Here's how the part is built. I have some questions about the finished solid (model axes, mm). Coordinates: 2 decimals unless noted, no trailing zeros. Write each loop counter-clockwise with the first axis right and the second up, starting at its lowest first coordinate (ties: lowest second). Pieces come first, ordered by that corner, then holes.
Item 1: If we section it at B-B (x = 35): Please give me the cut outline in (y, z).
Item 2: If I drill on line 1 (Y direction, x = 61, z = 51); line 2 (Z direction, x = 45, y = -67); line 3 (Z direction, x = 20, y = -56), over which ranges is the centre line in solid material (lowest first)?
Item 3: If we section it at A-A (y = -48.5): Please give me the cut outline in (x, z), then the cut area to 3 significant figures.
Item 4: I'm going to push flat-ended pins straight in: pin 1 Ø6 at (x, z) = (40, 60) entering from +Y; pin 2 Ø4 at (y, z) = (-12.5, 55) entering from +X; pin 3 Ø6 at (x, z) = (50.5, 33) entering from +Y; pin 4 Ø2 at (x, y) = (20, -33.5) entering from +Z. Where does each tip first touch, or does it pass through?
Item 5: If we section it at D-D (z = 11.5): Please give me the cut outline in (x, y).
Item 6: If we section it at C-C (z = 24): Please give me the cut outline in (x, y).
from build123d import *

# Parameters (mm, degrees)
F0_W     = 76.2
F0_H     = 76.2
F1_DEPTH = 76.2
F2_SIZE  = 25.4
F3_R     = 25.4


with BuildPart() as f1:
    # F0 (on Front) → F1 (new body)
    with BuildSketch(Plane.XZ):
        with Locations((38.1, 38.1)):
            Rectangle(F0_W, F0_H)
    extrude(amount=F1_DEPTH)

    # F2
    f2_edges = [f1.edges().sort_by_distance(p)[0] for p in [
        (0, -38.1, 0),
        (76.2, -38.1, 0),
        (38.1, 0, 0),
        (38.1, -76.2, 0),
    ]]
    chamfer(f2_edges, length=F2_SIZE)

    # F3
    f3_edges = [f1.edges().sort_by_distance(p)[0] for p in [
        (76.2, -38.1, 76.2),
        (0, -38.1, 76.2),
        (38.1, 0, 76.2),
        (38.1, -76.2, 76.2),
    ]]
    fillet(f3_edges, radius=F3_R)


solid = f1.part
Answer list:
1. outline: (-76.2, 25.4) - (-50.8, 0) - (-25.4, 0) - (0, 25.4) - (0, 50.8) arc R25.4 ccw to (-25.4, 76.2) - (-50.8, 76.2) arc R25.4 ccw to (-76.2, 50.8) - close
2. line 1: y = -76.2 to 0
2. line 2: z = 16.2 to 70.36
2. line 3: z = 5.4 to 75.62
3. outline: (0, 25.4) - (25.4, 0) - (50.8, 0) - (76.2, 25.4) - (76.2, 50.8) arc R25.4 ccw to (50.8, 76.2) - (25.4, 76.2) arc R25.4 ccw to (0, 50.8) - close
3. area: 4,880 mm2
4. pin 1: stops at y = -0.77
4. pin 2: stops at x = 76.1
4. pin 3: stops at y = 0
4. pin 4: stops at z = 75.82
5. outline: (13.9, -62.3) - (62.3, -62.3) - (62.3, -13.9) - (13.9, -13.9) - close
6. outline: (1.4, -74.8) - (74.8, -74.8) - (74.8, -1.4) - (1.4, -1.4) - close
